Could you check a few things on this model? Use its own coordinates, in mm. A direction names the side the tool comes from. Round coordinates to 2 decimals unless told otherwise and drop trailing zeros. Write each loop counter-clockwise with the first axis right and the second up, starting at its lowest first coordinate (ties: lowest second). Pieces come first, ordered by that corner, then holes.
```python
from build123d import *

# Parameters (mm, degrees)
ESBO_O1_W                        = 11.5
ESBO_O1_H                        = 12
RESSALTO_EXTRUS_O1_DEPTH         = 7
ESBO_O2_W                        = 10.5
ESBO_O2_H                        = 0.75
CORTE_EXTRUS_O1_DEPTH            = 13
ESBO_O3_W                        = 9.5
ESBO_O3_H                        = 12
RESSALTO_EXTRUS_O2_DEPTH         = 3.75
ESBO_O4_W                        = 7.5
ESBO_O4_H                        = 3
CORTE_EXTRUS_O2_DEPTH            = 13
ESBO_O5_W                        = 2
ESBO_O5_H                        = 0.4
RESSALTO_EXTRUS_O3_DEPTH         = 7
ESBO_O6_W                        = 0.5
ESBO_O6_H                        = 4
CORTE_EXTRUS_O3_DEPTH            = 9.7
ESBO_O7_W                        = 0.5
ESBO_O7_H                        = 4
CORTE_EXTRUS_O4_DEPTH            = 9.7
ESBO_O8_W                        = 4.75
ESBO_O8_H                        = 2
RESSALTO_EXTRUS_O4_DEPTH         = 3
ESBO_O9_W                        = 1
ESBO_O9_H                        = 0.75
CORTE_EXTRUS_O5_DEPTH            = 13
ESBO_O10_W                       = 2
ESBO_O10_H                       = 0.4
RESSALTO_EXTRUS_O5_DEPTH         = 3
ESBO_O11_W                       = 2
ESBO_O11_H                       = 0.4
RESSALTO_EXTRUS_O6_DEPTH         = 3
ESBO_O12_W                       = 2
ESBO_O12_H                       = 0.4
RESSALTO_EXTRUS_O7_DEPTH         = 3
ESBO_O13_W                       = 1
ESBO_O13_H                       = 0.4
RESSALTO_EXTRUS_O8_DEPTH         = 0.5
ESBO_O14_W                       = 0.75
ESBO_O14_H                       = 0.5
ESBO_O15_W                       = 0.75
ESBO_O15_H                       = 0.5
ESBO_O16_W                       = 3.5
ESBO_O16_H                       = 3.5
FURO_DE_DI_METRO_3_6_3_6_1_D     = 3.6
FURO_DE_DI_METRO_3_6_3_6_1_DEPTH = 3.5
CHANFRO1_SIZE                    = 0.3
ESBO_O19_W                       = 0.43
ESBO_O19_H                       = 1
RESSALTO_EXTRUS_O9_DEPTH         = 0.5
RESSALTO_EXTRUS_O10_DEPTH        = 0.5
RESSALTO_EXTRUS_O11_START        = -0.5
RESSALTO_EXTRUS_O11_DEPTH        = 1


with BuildPart() as part:
    # Esboço1 → Ressalto-extrusão1 (new body)
    with BuildSketch(Plane(origin=(0, 0, -3.5), x_dir=(-1, 0, 0), z_dir=(0, 0, -1))):
        with Locations((9.25, 0)):
            Rectangle(ESBO_O1_W, ESBO_O1_H)
    extrude(amount=-RESSALTO_EXTRUS_O1_DEPTH)

    # Esboço2 → Corte-extrusão1 (cut, through all)
    with BuildSketch(Plane(origin=(0, 6, 0), x_dir=(-1, 0, 0), z_dir=(0, 1, 0))):
        with Locations((9.75, -3.125)):
            Rectangle(ESBO_O2_W, ESBO_O2_H)
    extrude(amount=-CORTE_EXTRUS_O1_DEPTH, mode=Mode.SUBTRACT)

    # Esboço3 → Ressalto-extrusão2 (add)
    with BuildSketch(Plane(origin=(0, 0, -2.75), x_dir=(-1, 0, 0), z_dir=(0, 0, -1))):
        with Locations((10.25, 0)):
            Rectangle(ESBO_O3_W, ESBO_O3_H)
    extrude(amount=RESSALTO_EXTRUS_O2_DEPTH)

    # Esboço4 → Corte-extrusão2 (cut, through all)
    with BuildSketch(Plane.XZ.offset(6)):
        with Locations((-11.25, -5)):
            Rectangle(ESBO_O4_W, ESBO_O4_H)
    extrude(amount=-CORTE_EXTRUS_O2_DEPTH, mode=Mode.SUBTRACT)

    # Esboço5 → Ressalto-extrusão3 (add)
    with BuildSketch(Plane(origin=(0, 0, -3.5), x_dir=(-1, 0, 0), z_dir=(0, 0, -1))):
        with Locations((11.5, -2.5)):
            Rectangle(ESBO_O5_W, ESBO_O5_H)
    extrude(amount=RESSALTO_EXTRUS_O3_DEPTH)

    # Esboço6 → Corte-extrusão3 (cut, through all)
    with BuildSketch(Plane.XZ.offset(2.7)):
        with Locations((-10.75, -8.5)):
            Rectangle(ESBO_O6_W, ESBO_O6_H)
    extrude(amount=-CORTE_EXTRUS_O3_DEPTH, mode=Mode.SUBTRACT)

    # Esboço7 → Corte-extrusão4 (cut, through all)
    with BuildSketch(Plane.XZ.offset(2.7)):
        with Locations((-12.25, -8.5)):
            Rectangle(ESBO_O7_W, ESBO_O7_H)
    extrude(amount=-CORTE_EXTRUS_O4_DEPTH, mode=Mode.SUBTRACT)

    # Esboço8 → Ressalto-extrusão4 (add)
    with BuildSketch(Plane(origin=(0, 0, -3.5), x_dir=(-1, 0, 0), z_dir=(0, 0, -1))):
        with Locations((9.875, 0)):
            Rectangle(ESBO_O8_W, ESBO_O8_H)
    extrude(amount=RESSALTO_EXTRUS_O4_DEPTH)

    # Esboço9 → Corte-extrusão5 (cut, through all)
    with BuildSketch(Plane.XZ.offset(6)):
        with Locations((-5, 3.125)):
            Rectangle(ESBO_O9_W, ESBO_O9_H)
    extrude(amount=-CORTE_EXTRUS_O5_DEPTH, mode=Mode.SUBTRACT)

    # Esboço10 → Ressalto-extrusão5 (add)
    with BuildSketch(Plane(origin=(0, 0, -3.5), x_dir=(-1, 0, 0), z_dir=(0, 0, -1))):
        with Locations((11.5, 5)):
            Rectangle(ESBO_O10_W, ESBO_O10_H)
    extrude(amount=RESSALTO_EXTRUS_O5_DEPTH)

    # Esboço11 → Ressalto-extrusão6 (add)
    with BuildSketch(Plane(origin=(0, 0, -3.5), x_dir=(-1, 0, 0), z_dir=(0, 0, -1))):
        with Locations((11.5, -5)):
            Rectangle(ESBO_O11_W, ESBO_O11_H)
    extrude(amount=RESSALTO_EXTRUS_O6_DEPTH)

    # Esboço12 → Ressalto-extrusão7 (add)
    with BuildSketch(Plane(origin=(0, 0, -3.5), x_dir=(-1, 0, 0), z_dir=(0, 0, -1))):
        with Locations((11.5, 2.5)):
            Rectangle(ESBO_O12_W, ESBO_O12_H)
    extrude(amount=RESSALTO_EXTRUS_O7_DEPTH)

    # Esboço13 → Ressalto-extrusão8 (add)
    with BuildSketch(Plane(origin=(0, 0, -6.5), x_dir=(-1, 0, 0), z_dir=(0, 0, -1))):
        with Locations((11.5, 0)):
            Rectangle(ESBO_O13_W, ESBO_O13_H)
    extrude(amount=RESSALTO_EXTRUS_O8_DEPTH)

    # Esboço14 → Revolução1 (revolve)
    with BuildSketch(Plane(origin=(0, -5, 0), x_dir=(1, 0, 0), z_dir=(0, 1, 0))):
        with Locations((-6.125, 6.75)):
            Rectangle(ESBO_O14_W, ESBO_O14_H)
    revolve(axis=Axis((-6.5, -5, -7), (0, 0, 1)))

    # Esboço15 → Revolução2 (revolve)
    with BuildSketch(Plane(origin=(0, 5, 0), x_dir=(1, 0, 0), z_dir=(0, 1, 0))):
        with Locations((-6.125, 6.75)):
            Rectangle(ESBO_O15_W, ESBO_O15_H)
    revolve(axis=Axis((-6.5, 5, -7), (0, 0, 1)))

    # Esboço16 → Revolução3 (revolve)
    with BuildSketch(Plane(origin=(0, 0, 0), x_dir=(-1, 0, 0), z_dir=(0, 0, -1))):
        with Locations((1.75, 1.75)):
            Rectangle(ESBO_O16_W, ESBO_O16_H)
    revolve(axis=Axis((0, 0, 0), (-1, 0, 0)))

    # Furo de diâmetro Ø3.6 (3.6)1
    with Locations(Plane(origin=(0, 0, 0), x_dir=(0, 0, -1), z_dir=(1, 0, 0))):
        with Locations((0, 0)):
            Hole(FURO_DE_DI_METRO_3_6_3_6_1_D / 2, depth=FURO_DE_DI_METRO_3_6_3_6_1_DEPTH)

    # Chanfro1
    chanfro1_edges = [part.edges().sort_by_distance(p)[0] for p in [
        (0, -3.5, 0),
    ]]
    chamfer(chanfro1_edges, length=CHANFRO1_SIZE)

    # Esboço19 → Ressalto-extrusão9 (add)
    with BuildSketch(Plane(origin=(0, 0, -6.5), x_dir=(-1, 0, 0), z_dir=(0, 0, -1))):
        with Locations((6.505, 0)):
            Rectangle(ESBO_O19_W, ESBO_O19_H)
    extrude(amount=RESSALTO_EXTRUS_O9_DEPTH)

    # Esboço20 → Ressalto-extrusão10 (add, symmetric)
    with BuildSketch(Plane(origin=(0, 0, 0), x_dir=(1, 0, 0), z_dir=(0, 1, 0))):
        Polygon((-6.302158206, 6.98750552), (-5.732158206, 9.13750552), (-6.352158206, 10.73750552), (-6.713447386, 10.597505963), (-6.147697214, 9.13750552), (-6.717697214, 6.98750552), align=None)
    extrude(amount=RESSALTO_EXTRUS_O10_DEPTH, both=True)

    # Esboço21 → Ressalto-extrusão11 (add)
    with BuildSketch(Plane.ZY.offset(12.5).offset(RESSALTO_EXTRUS_O11_START)):
        Polygon((-6.5, 5.2), (-8.9, 5.86), (-10.5, 5.2), (-10.35899319, 4.858165309), (-8.9, 5.46), (-6.5, 4.8), align=None)
    ressalto_extrus_o11 = extrude(amount=-RESSALTO_EXTRUS_O11_DEPTH)

    # Espelhar1: Ressalto-extrusão11 across plane
    add(ressalto_extrus_o11.mirror(Plane.ZX))


solid = part.part
```
Q1. I'm going to push flat-ended pins straight in: pin 1 Ø1.5 at (y, z) = (0.5, -3.5) entering from +X; pin 2 Ø0.9 at (y, z) = (-2.5, -5) entering from -X; pin 3 Ø4 at (x, y) = (-6, 4) entering from -Z; pin 4 Ø0.6 at (y, z) = (0, -6.5) entering from -X. Where does each tip first touch, or does it pass through?
Q2. On a 3-axis mill with a long thin cutter (end or side, diameter ignored), from which of +Z, -Z, +X, -X, +Y, -Y can I reach the whole of each face in a straight line? I mean faces 4 (the flat face through (-11, 5.2, -5)), 5 (the flat face through (-10, 1, -5)), 6 (the flat face through (-6.435, 0.007, -9.878)), 7 (the cylindrical face through (-7.095, 4.544, -6.754)). Say none if no direction works.
Q3. If I drill on L1, parallel to Y at x = -0.85, z = 0; L2, parallel to X at y = -4.5, z = 3.25; L3, parallel to X at y = -4, z = -2, over which ranges is the centre line in solid material (lowest first)?
Q4. We'd pull the mould along X, two halves only. Please class faces 1 (the cylindrical face through (-1.774, 0.541, 1.717)), 2 (the flat face through (-3.5, -4, 0)), 3 (the flat face through (-5, 0, -2.75)): pulls with the +X half, pulls with the -X half, needs draft (parallel to the pull), parting line crosses it, or undercut.
Q5. Imagine slicing it at B-B, the plane y = 3.75. Write out the boundary of the cut face in (x, z).
Q6. Imagine slicing it at C-C, the plane z = -7.75. Write out the boundary of the cut face in (x, y).
Q7. Imagine slicing it at D-D, the plane x = -1. Write out the boundary of the cut face in (y, z), then the cut area to 3 significant figures.
Q8. Imagine slicing it at A-A, the plane x = -8.75. Write out the boundary of the cut face in (y, z), then the cut area to 3 significant figures.
Results found:
1. pin 1: stops at x = 0
1. pin 2: stops at x = -12.5
1. pin 3: stops at z = -7
1. pin 4: stops at x = -12.25
2. face 4: -X, +Y
2. face 5: -Z, -X
2. face 6: -X, +Y, -Y
2. face 7: -Z
3. L1: y = -3.5 to -1.8, 1.8 to 3.5
3. L2: x = -15 to -5.5, -4.5 to -3.5
3. L3: x = -15 to -3.5
4. face 1: needs draft
4. face 2: pulls with the +X half
4. face 3: undercut
5. outline: (-15, -3.5) - (-7.5, -3.5) - (-7.5, -6.5) - (-5.5, -6.5) - (-5.5, -2.75) - (-4.5, -2.75) - (-4.5, -3.5) - (-3.5, -3.5) - (-3.5, 3.5) - (-4.5, 3.5) - (-4.5, 2.75) - (-5.5, 2.75) - (-5.5, 3.5) - (-15, 3.5) - close
6. outline: (-12, -5.54) - (-11, -5.54) - (-11, -5.14) - (-12, -5.14) - close; (-12, -2.7) - (-11, -2.7) - (-11, -2.3) - (-12, -2.3) - close; (-12, 5.14) - (-11, 5.14) - (-11, 5.54) - (-12, 5.54) - close; (-6.52, -0.5) - (-6.1, -0.5) - (-6.1, 0.5) - (-6.52, 0.5) - close
7. outline: circle Ø7 at (0, 0); hole circle Ø3.6 at (0, 0)
7. area: 28.3 mm2
8. outline: (-6, -3.5) - (-1, -3.5) - (-1, -6.5) - (1, -6.5) - (1, -3.5) - (6, -3.5) - (6, 3.5) - (-6, 3.5) - close
8. area: 90.0 mm2
